from build123d import *

# Parameters (mm, degrees)
PAD001_DEPTH    = 0.2
CHAMFER001_SIZE = 0.5
SKETCH002_W     = 8
SKETCH002_H     = 3.86
PAD002_DEPTH    = 0.2
PAD004_DEPTH    = 4.98
PAD003_DEPTH    = 4.98
PAD_DEPTH       = 0.2
CHAMFER_SIZE    = 0.5
FILLET_R        = 0.4
FILLET001_R     = 0.19


with BuildPart() as body001:
    # Sketch001 → Pad001 (new body)
    with BuildSketch(Plane.XY.offset(3.66)):
        Polygon((0, 0), (1.57, 0), (1.57, 3.18), (2.18, 3.18), (2.18, 11.18), (1.37, 11.18), (1.37, 6.2), (0, 6.2), align=None)
    extrude(amount=PAD001_DEPTH)

    # Chamfer001
    chamfer001_edges = [body001.edges().sort_by_distance(p)[0] for p in [
        (1.57, 0, 3.76),
        (0, 0, 3.76),
    ]]
    chamfer(chamfer001_edges, length=CHAMFER001_SIZE)

    # Sketch002 (on Face11 of Chamfer001) → Pad002 (join)
    with BuildSketch(Plane.YZ.offset(2.18)):
        with Locations((7.18, 1.93)):
            Rectangle(SKETCH002_W, SKETCH002_H)
    extrude(amount=-PAD002_DEPTH)


with BuildPart() as body003:
    # Sketch004 → Pad004 (new body)
    with BuildSketch(Plane.XZ):
        with BuildLine():
            Line((1.37, 0.2), (1.37, 0))
            ThreePointArc((1.37, 1.6), (0.57, 0.8), (1.37, 0))
            Line((1.37, 1.6), (1.37, 1.4))
            ThreePointArc((1.37, 1.4), (0.77, 0.8), (1.37, 0.2))
        make_face()
    extrude(amount=PAD004_DEPTH)


with BuildPart() as body003_1:
    # Body003 placement: moved
    add(body003.part.moved(Location((0, 11.18, 2.25))))


with BuildPart() as body002:
    # Sketch003 → Pad003 (new body)
    with BuildSketch(Plane.XZ):
        with BuildLine():
            Line((1.37, 0.2), (1.37, 0))
            ThreePointArc((1.37, 1.6), (0.57, 0.8), (1.37, 0))
            Line((1.37, 1.6), (1.37, 1.4))
            ThreePointArc((1.37, 1.4), (0.77, 0.8), (1.37, 0.2))
        make_face()
    extrude(amount=PAD003_DEPTH)


with BuildPart() as body002_1:
    # Body002 placement: moved
    add(body002.part.moved(Location((0, 11.18, 0))))


with BuildPart() as body:
    # Sketch → Pad (new body)
    with BuildSketch(Plane.XY):
        Polygon((0, 0), (1.57, 0), (1.57, 3.18), (2.18, 3.18), (2.18, 11.18), (1.37, 11.18), (1.37, 6.2), (0, 6.2), align=None)
    extrude(amount=PAD_DEPTH)

    # Chamfer
    chamfer_edges = [body.edges().sort_by_distance(p)[0] for p in [
        (1.57, 0, 0.1),
        (0, 0, 0.1),
    ]]
    chamfer(chamfer_edges, length=CHAMFER_SIZE)

    # Boolean: union Body001, Body003, Body002
    add(body001.part)
    add(body003_1.part)
    add(body002_1.part)

    # Fillet
    fillet_edges = [body.edges().sort_by_distance(p)[0] for p in [
        (1.98, 7.18, 0.2),
        (1.98, 7.18, 3.66),
    ]]
    fillet(fillet_edges, radius=FILLET_R)

    # Fillet001
    fillet001_edges = [body.edges().sort_by_distance(p)[0] for p in [
        (2.18, 7.18, 0),
        (2.18, 7.18, 3.86),
    ]]
    fillet(fillet001_edges, radius=FILLET001_R)


solid = body.part
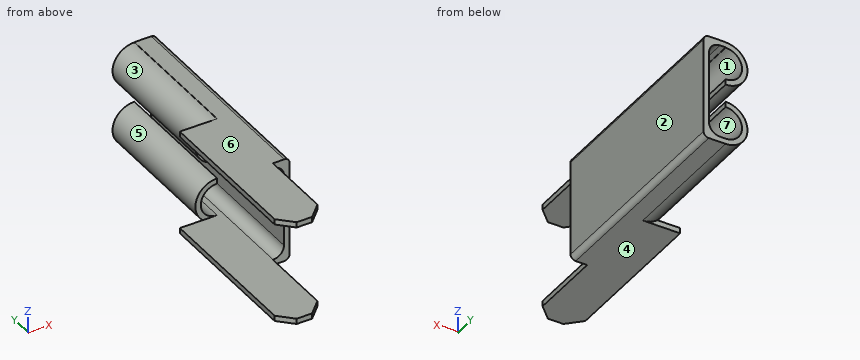
Geometry: final body of the model. Coordinates: model frame, mm. Face numbers are marked on the shaded views. A direction names the side the tool comes from. Give positions to 0.01 mm unless a question says otherwise; leave off trailing zeros. Order: outer loops, then holes, each group sorted by start corner. A loop starts at its lowest first (then second) coordinate and runs counter-clockwise, first axis right, second up. Notation, with made-up numbers: (-27.75, 14.5) -> (-10.75, 14.5) arc R30 ccw to (-10.75, 45.5) -> close; hole circle Ø5 at (22, 38.25). An arc over 180 degrees is marked (long way). Answer as a JSON object with one key per item and string values.
Q1. Access query for the marked faces 1, 2 and 3. Directions: +Z, -Z, +X, -X, +Y, -Y. A direction counts if a zero-diameter tool reaches every point of the face in a straight line with its end or side. Return the directions, or none.
Entries:
{"face 1": "+Y, -Y", "face 2": "+Z, -Z, +X, +Y, -Y", "face 3": "-X, +Y"}
Q2. Section C-C (x = 1.8). Output: boundary loops of the cut face in (y, z), plus the area to 3 significant figures.
Entries:
{"outline": "(3.18, 0) -> (11.18, 0) -> (11.18, 0.27) -> (3.18, 0.27) -> close; (3.18, 3.59) -> (11.18, 3.59) -> (11.18, 3.86) -> (3.18, 3.86) -> close", "area": "4.25 mm^2"}
Q3. Material intervals for probe 1 along X at (y, z) = (7.5, 3.05); probe 2 along Z at (x, y) = (1.6, 6.75); probe 3 along Y at (x, z) = (0.7, 0.6), sorted ascending.
Entries:
{"probe 1": "x = 0.57 to 0.77, 1.98 to 2.18", "probe 2": "z = 0 to 0.2, 3.66 to 3.86", "probe 3": "y = 6.2 to 11.18"}
Q4. First-contact query: pin 1 (0.8 mm diameter, centred on x = 1, y = 6.5, fed in from -Z); pin 2 (2 mm diameter, centred on y = 8, z = 2, fed in from -X); pin 3 (0.7 mm diameter, centred on x = 2, z = 1.5, fed in from -Y). Flat tips, straight axial feed; report the tip coordinate or a pass-through.
Entries:
{"pin 1": "stops at z = 0", "pin 2": "stops at x = 0.57", "pin 3": "stops at y = 3.18"}
Q5. Draft query along Z for the marked faces 4, 5, 6 and 7. Return one class per face: released by +Z, released by -Z, zero draft, split by the parting line, or undercut.
Entries:
{"face 4": "released by -Z", "face 5": "undercut", "face 6": "released by +Z", "face 7": "undercut"}
Q6. Section D-D (x = 0.95). Output: boundary loops of the cut face in (y, z), plus the area to 3 significant figures.
Entries:
{"outline": "(0, 0) -> (6.2, 0) -> (6.2, 0.12) -> (11.18, 0.12) -> (11.18, 0.37) -> (6.2, 0.37) -> (6.2, 0.2) -> (0, 0.2) -> close; (0, 3.66) -> (6.2, 3.66) -> (6.2, 3.48) -> (11.18, 3.48) -> (11.18, 3.73) -> (6.2, 3.73) -> (6.2, 3.86) -> (0, 3.86) -> close; (6.2, 1.23) -> (11.18, 1.23) -> (11.18, 1.48) -> (6.2, 1.48) -> close; (6.2, 2.37) -> (11.18, 2.37) -> (11.18, 2.62) -> (6.2, 2.62) -> close", "area": "7.51 mm^2"}
Q7. Section A-A (z = 0.8). Output: boundary loops of the cut face in (x, y), plus the area to 3 significant figures.
Entries:
{"outline": "(0.57, 6.2) -> (0.77, 6.2) -> (0.77, 11.18) -> (0.57, 11.18) -> close; (1.98, 3.18) -> (2.18, 3.18) -> (2.18, 11.18) -> (1.98, 11.18) -> close", "area": "2.60 mm^2"}
